```python
from build123d import *

# Parameters (mm, degrees)
SKETCH_W        = 100
SKETCH_H        = 64
SKETCH_R        = 3.2
SKETCH_R_2      = 1.8
SKETCH_R_3      = 4
PAD_DEPTH       = 15
SKETCH001_R     = 11.2
SKETCH001_R_2   = 6
POCKET_DEPTH    = 5.4
SKETCH002_R     = 3.2
POCKET001_DEPTH = 3.2
SKETCH003_R     = 6
POCKET002_DEPTH = 5.4
SKETCH004_R     = 3.2
POCKET003_DEPTH = 15
FILLET_R        = 2


with BuildPart() as part:
    # Sketch → Pad (new body)
    with BuildSketch(Plane.XY):
        with Locations((50, 32)):
            Rectangle(SKETCH_W, SKETCH_H)
        with Locations((50, 42.85)):
            Circle(SKETCH_R, mode=Mode.SUBTRACT)
        with Locations((65.5, 58.35)):
            Circle(SKETCH_R_2, mode=Mode.SUBTRACT)
        with Locations((65.5, 27.35)):
            Circle(SKETCH_R_2, mode=Mode.SUBTRACT)
        with Locations((34.5, 27.35)):
            Circle(SKETCH_R_2, mode=Mode.SUBTRACT)
        with Locations((34.5, 58.35)):
            Circle(SKETCH_R_2, mode=Mode.SUBTRACT)
        with Locations((20, 10)):
            Circle(SKETCH_R, mode=Mode.SUBTRACT)
        with Locations((80, 10)):
            Circle(SKETCH_R, mode=Mode.SUBTRACT)
        with Locations((82, 42.85)):
            Circle(SKETCH_R_3, mode=Mode.SUBTRACT)
        with Locations((18, 42.85)):
            Circle(SKETCH_R_3, mode=Mode.SUBTRACT)
    extrude(amount=PAD_DEPTH)

    # Sketch001 (on Face15 of Pad) → Pocket (cut)
    with BuildSketch(Plane.XY.offset(15)):
        with Locations((50, 42.85)):
            Circle(SKETCH001_R)
        with Locations((20, 10)):
            Circle(SKETCH001_R_2)
        with Locations((80, 10)):
            Circle(SKETCH001_R_2)
    extrude(amount=-POCKET_DEPTH, mode=Mode.SUBTRACT)

    # Sketch002 (on Face4 of Pocket) → Pocket001 (cut)
    with BuildSketch(Plane(origin=(0, 0, 0), x_dir=(1, 0, 0), z_dir=(0, 0, -1))):
        with Locations((34.5, -27.35)):
            Circle(SKETCH002_R)
        with Locations((65.5, -27.35)):
            Circle(SKETCH002_R)
        with Locations((34.5, -58.35)):
            Circle(SKETCH002_R)
        with Locations((65.5, -58.35)):
            Circle(SKETCH002_R)
    extrude(amount=-POCKET001_DEPTH, mode=Mode.SUBTRACT)

    # Sketch003 (on Face5 of Pocket001) → Pocket002 (cut)
    with BuildSketch(Plane.XY.offset(15)):
        with Locations((40, 10)):
            Circle(SKETCH003_R)
        with Locations((60, 10)):
            Circle(SKETCH003_R)
    extrude(amount=-POCKET002_DEPTH, mode=Mode.SUBTRACT)

    # Sketch004 (on Face4 of Pocket002) → Pocket003 (cut)
    with BuildSketch(Plane(origin=(0, 0, 0), x_dir=(1, 0, 0), z_dir=(0, 0, -1))):
        with Locations((40, -10)):
            Circle(SKETCH004_R)
        with Locations((60, -10)):
            Circle(SKETCH004_R)
    extrude(amount=-POCKET003_DEPTH, mode=Mode.SUBTRACT)

    # Fillet
    fillet_edges = [part.edges().sort_by_distance(p)[0] for p in [
        (0, 64, 7.5),
        (100, 64, 7.5),
        (100, 0, 7.5),
        (0, 0, 7.5),
    ]]
    fillet(fillet_edges, radius=FILLET_R)


solid = part.part
```
Could you check a few things on this model? Use its own coordinates, in mm. A direction names the side the tool comes from. Coordinates: 2 decimals unless noted, no trailing zeros. Order: outer loops, then holes, each group sorted by start corner. A loop starts at its lowest first (then second) coordinate and runs counter-clockwise, first axis right, second up. Notation, with made-up numbers: M 79.25,9 L 109.25,9 A8 cw 109.25,19 Z; hole C -13.75,32 d1. An arc over 180 degrees is marked long. Use one line per item in the form item = value. Start each with the question number.
1. Suppose I cut it at C-C on z = 7. Count the separate pieces of the cut face and the enclosed holes in it, then the cut area to 3 significant figures.
2. Suppose I cut it at D-D on y = 42.85. Write out the boundary of the cut face in (x, z).
3. On a 3-axis mill with a long thin cutter (end or side, diameter ignored), from which of +Z, -Z, +X, -X, +Y, -Y can I reach the whole of each face in a straight line? I mean faces 1 (the cylindrical face through (22.769, 4.677, 12.338)), 2 (the flat face through (49, 32, 0)), 3 (the flat face through (36, 29, 3.2)). Say none if no direction works.
4. For pin 1 (4.5 mm diameter, centred on x = 34.5, y = 27.35, fed in from -Z); pin 2 (7 mm diameter, centred on x = 80, y = 10, fed in from +Z), each with a flat end and sliding along its axis, tell me the tip position at first contact or that it passes through.
5. Please list where these lines run through material, in increasing order: line 1 (X direction, y = 58.35, z = 0.7); line 2 (X direction, y = 27.5, z = 7.5); line 3 (X direction, y = 10, z = 2.5).
6. Suppose I cut it at A-A on y = 58.35. Write out the boundary of the cut face in (x, z), then the cut area to 3 significant figures.
7. Suppose I cut it at B-B on x = 65. Write out the boundary of the cut face in (y, z), then the cut area to 3 significant figures.
8. We'd pull the mould along X, two halves only. Please class faces 4 (the flat face through (49, 64, 7)), 5 (the flat face through (23, 7, 9.6)), 6 (the cylindrical face through (99.4, 63.43, 7.6)), 7 (the flat face through (36, 60, 3.2)): +X half, -X half, draft (parallel to the pull), parting line (faces both ways), or undercut.
Geometry says:
q1.separate_pieces = 1
q1.enclosed_holes = 11
q1.area = 6,090 mm^2
q2.outline = M 0,0 L 14,0 L 14,15 L 0,15 Z; M 22,0 L 46.8,0 L 46.8,9.6 L 38.8,9.6 L 38.8,15 L 22,15 Z; M 53.2,0 L 78,0 L 78,15 L 61.2,15 L 61.2,9.6 L 53.2,9.6 Z; M 86,0 L 100,0 L 100,15 L 86,15 Z
q3.face_1 = +Z
q3.face_2 = -Z, +X, -X, +Y, -Y
q3.face_3 = -Z
q4.pin_1 = 3.2
q4.pin_2 = 9.6
q5.line_1 = 0 to 31.3, 37.7 to 62.3, 68.7 to 100
q5.line_2 = 0 to 32.71, 36.29 to 63.71, 67.29 to 100
q5.line_3 = 0 to 16.8, 23.2 to 36.8, 43.2 to 56.8, 63.2 to 76.8, 83.2 to 100
q6.outline = M 0,0 L 31.3,0 L 31.3,3.2 L 32.7,3.2 L 32.7,15 L 0,15 Z; M 36.3,3.2 L 37.7,3.2 L 37.7,0 L 62.3,0 L 62.3,3.2 L 63.7,3.2 L 63.7,15 L 36.3,15 Z; M 67.3,3.2 L 68.7,3.2 L 68.7,0 L 100,0 L 100,15 L 67.3,15 Z
q6.area = 1,370 mm^2
q7.outline = M 0,0 L 24.19,0 L 24.19,3.2 L 25.62,3.2 L 25.62,15 L 13.32,15 L 13.32,9.6 L 6.68,9.6 L 6.68,15 L 0,15 Z; M 29.08,3.2 L 30.51,3.2 L 30.51,0 L 55.19,0 L 55.19,3.2 L 56.62,3.2 L 56.62,15 L 29.08,15 Z; M 60.08,3.2 L 61.51,3.2 L 61.51,0 L 64,0 L 64,15 L 60.08,15 Z
q7.area = 802 mm^2
q8.face_4 = draft
q8.face_5 = undercut
q8.face_6 = +X half
q8.face_7 = undercut
